CAD build for the part. Positions are in the model's coordinates, mm. Face numbers are marked on the shaded views. A direction names the side the tool comes from. Coordinates: 2 decimals unless noted, no trailing zeros. Loops run counter-clockwise (first coordinate to the right, second up) from the corner with the lowest first, then second, coordinate; pieces in that order, holes last. Notation, with made-up numbers: (55, 64) -> (83, 64) arc R33 cw to (83, 96) -> close; hole circle Ø4 at (77, 76). An arc over 180 degrees is marked (long way). Write item = value, one per line. Start each with the question number.
(1) Drill centre lines: line 1 (X direction, y = 5.5, z = 0); line 2 (Y direction, x = -6.75, z = 0); line 3 (X direction, y = 7.75, z = 2.25). Where is each one in solid material? Low to high. Write a range as from..to.
(2) Band-saw the part on B-B (x = 0). Write the cut outline in (y, z).
(3) Band-saw the part on D-D (x = -5). Write the cut outline in (y, z).
(4) Flat gauge pins, fed straight in: P1, Ø2, axis at x = 7, z = 5, coming from the -Y side; P2, Ø3, axis at x = -0.5, y = 5, coming from the +Z side. Where does each tip first touch, or does it go through?
(5) Band-saw the part on A-A (z = 0). Write the cut outline in (x, y).
(6) Tool access for the marked faces 5, 6 and 7: list every direction of +Z, -Z, +X, -X, +Y, -Y with a clear straight run to the whole face (end or side of a thin tool).
(7) Pull direction Z, two halves, no side cores. Call the marked faces 1, 2, 3 and 4: +Z half, -Z half, draft (parallel to the pull), parting line (faces both ways), or undercut.
(8) Band-saw the part on C-C (y = 4.25). Write the cut outline in (x, z).
```python
from build123d import *

# Parameters (mm, degrees)
BOSS_EXTRUDE1_DEPTH = 10
SKETCH2_R           = 4.25
CUT_EXTRUDE1_DEPTH  = 9
BOSS_EXTRUDE2_START = -2
SKETCH3_R           = 9
BOSS_EXTRUDE2_DEPTH = 2


with BuildPart() as part:
    # Sketch1 → Boss-Extrude1 (new body)
    with BuildSketch(Plane(origin=(0, 0, 0), x_dir=(1, 0, 0), z_dir=(0, 1, 0))):
        with BuildLine():
            Line((1.802775638, -5), (-1.802775638, -5))
            ThreePointArc((-1.802775638, -5), (-2.337298122, -4.927248223), (-2.832933145, -4.714285714))
            ThreePointArc((-2.832933145, -4.714285714), (0, 5.5), (2.832933145, -4.714285714))
            ThreePointArc((2.832933145, -4.714285714), (2.337298122, -4.927248223), (1.802775638, -5))
        make_face()
    extrude(amount=BOSS_EXTRUDE1_DEPTH)

    # Sketch2 → Cut-Extrude1 (cut)
    with BuildSketch(Plane(origin=(0, 10, 0), x_dir=(1, 0, 0), z_dir=(0, 1, 0))):
        with Locations(Location((0, 0, 0), (0, 0, 270))):
            Circle(SKETCH2_R)
    extrude(amount=-CUT_EXTRUDE1_DEPTH, mode=Mode.SUBTRACT)

    # Sketch3 → Boss-Extrude2 (add)
    with BuildSketch(Plane(origin=(0, 10, 0), x_dir=(1, 0, 0), z_dir=(0, 1, 0)).offset(BOSS_EXTRUDE2_START)):
        with Locations(Location((0, 0, 0), (0, 0, 270))):
            Circle(SKETCH3_R)
        with BuildLine():
            Line((1.802775638, -5), (-1.802775638, -5))
            ThreePointArc((-1.802775638, -5), (-2.337298122, -4.927248223), (-2.832933145, -4.714285714))
            ThreePointArc((-2.832933145, -4.714285714), (0, 5.5), (2.832933145, -4.714285714))
            ThreePointArc((2.832933145, -4.714285714), (2.337298122, -4.927248223), (1.802775638, -5))
        make_face(mode=Mode.SUBTRACT)
    extrude(amount=BOSS_EXTRUDE2_DEPTH)


solid = part.part
```
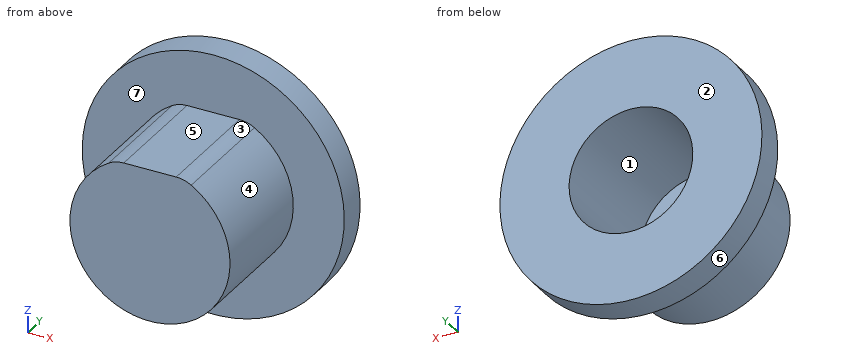
Findings below:
q1.line_1 = -5.5..-4.25, 4.25..5.5
q1.line_2 = 8..10
q1.line_3 = -5.02..-3.61, 3.61..5.02
q2.outline = (0, -5.5) -> (8, -5.5) -> (8, -9) -> (10, -9) -> (10, -4.25) -> (1, -4.25) -> (1, 4.25) -> (10, 4.25) -> (10, 9) -> (8, 9) -> (8, 5) -> (0, 5) -> close
q3.outline = (0, -2.29) -> (8, -2.29) -> (8, -7.48) -> (10, -7.48) -> (10, 7.48) -> (8, 7.48) -> (8, 2.29) -> (0, 2.29) -> close
q4.P1 = 8
q4.P2 = 5
q5.outline = (-9, 8) -> (-5.5, 8) -> (-5.5, 0) -> (5.5, 0) -> (5.5, 8) -> (9, 8) -> (9, 10) -> (4.25, 10) -> (4.25, 1) -> (-4.25, 1) -> (-4.25, 10) -> (-9, 10) -> close
q6.face_5 = +Z, +X, -X, -Y
q6.face_6 = +Y, -Y
q6.face_7 = -Y
q7.face_1 = undercut
q7.face_2 = draft
q7.face_3 = +Z half
q7.face_4 = parting line
q8.outline = (-2.83, 4.71) arc R5.5 ccw (long way) to (2.83, 4.71) arc R2 ccw to (1.8, 5) -> (-1.8, 5) arc R2 ccw to start; hole circle Ø8.5 at (0, 0)
